```python
from build123d import *

# Parameters (mm, degrees)
CROQUIS1_R              = 9.25
SALIENTE_EXTRUIR1_DEPTH = 5
CROQUIS1_6_R            = 4.5
CROQUIS1_6_R_2          = 3
EXTRUIR_L_MINA1_DEPTH   = 35


with BuildPart() as part:
    # Croquis1 → Saliente-Extruir1 (new body)
    with BuildSketch(Plane.XY):
        Circle(CROQUIS1_R)
    extrude(amount=SALIENTE_EXTRUIR1_DEPTH)

    # Croquis1<6> → Extruir-Lámina1 (add)
    with BuildSketch(Plane.XY):
        Circle(CROQUIS1_6_R)
        Circle(CROQUIS1_6_R_2, mode=Mode.SUBTRACT)
    extrude(amount=EXTRUIR_L_MINA1_DEPTH)


solid = part.part
```
Build history of the part. All positions in model axes, mm. A direction names the side the tool comes from. Round coordinates to 2 decimals unless told otherwise and drop trailing zeros. Write each loop counter-clockwise with the first axis right and the second up, starting at its lowest first coordinate (ties: lowest second). Pieces come first, ordered by that corner, then holes. Notation, with made-up numbers: (-22, 12.5) -> (26, 12.5) arc R7 cw to (26, 23.5) -> close; hole circle Ø3 at (76.25, 21.5). An arc over 180 degrees is marked (long way). Put each result on its own line as item: value.
Item 1: Slice it at A-A, the plane x = 0. Give the cut face in (y, z), plus the area to 4 significant figures.
Here are the results:
outline: (-9.25, 0) -> (9.25, 0) -> (9.25, 5) -> (4.5, 5) -> (4.5, 35) -> (3, 35) -> (3, 5) -> (-3, 5) -> (-3, 35) -> (-4.5, 35) -> (-4.5, 5) -> (-9.25, 5) -> close
area: 182.5 mm^2
Item 2: Tool access for faces 4 (the face through (1, -3, 35)), 5 (the face through (-3, 0, 20)): list every direction of +Z, -Z, +X, -X, +Y, -Y with a clear straight run to the whole face (end or side of a thin tool).
Here are the results:
face 4: +Z, +X, -X, +Y, -Y
face 5: +Z
Item 3: Wall check: probe 1 along Y at (x, z) = (0, 13.5); probe 2 along Z at (x, y) = (-5, -1). Give the ranges that are in metal, low to high. Write a range as from..to.
Here are the results:
probe 1: y = -4.5..-3, 3..4.5
probe 2: z = 0..5
Item 4: Slice it at C-C, the plane z = 4. Give the cut face in (x, y), plus the area to 3 significant figures.
Here are the results:
outline: circle Ø18.5 at (0, 0)
area: 269 mm^2
Item 5: Slice it at D-D, the plane z = 29.5. Give the cut face in (x, y), plus the area to 3 significant figures.
Here are the results:
outline: circle Ø9 at (0, 0); hole circle Ø6 at (0, 0)
area: 35.3 mm^2
Item 6: Two-plate mould, pull along X, no slides. Class faces 1 (the face through (0, 0, 0)), 2 (the face through (-0.59, 4.46, 19.79)), 3 (the face through (0, 0, 5)): pulls with the +X half, pulls with the -X half, needs draft (parallel to the pull), parting line crosses it, or undercut.
Here are the results:
face 1: needs draft
face 2: parting line crosses it
face 3: undercut
Item 7: Flat gauge pins, fed straight in: P1, Ø4, axis at x = 7, y = 2, coming from the +Z side; P2, Ø8, axis at x = 0, y = 0, coming from the +Z side; P3, Ø5, axis at x = 4, z = 18, coming from the +Y side; P4, Ø5, axis at x = 2, z = 10.5, coming from the +Y side. Where does each tip first touch, or does it go through?
Here are the results:
P1: stops at z = 5
P2: stops at z = 35
P3: stops at y = 4.24
P4: stops at y = 4.5
